Study the drawing (mm; zero at the part's minimum x, y, z) and answer. Coordinates: 2 decimals unless noted, no trailing zeros. Loops run counter-clockwise (first coordinate to the right, second up) from the corner with the lowest first, then second, coordinate; pieces in that order, holes last. Notation, with made-up numbers: (53.25, 40.5) -> (69.25, 40.5) arc R19 cw to (69.25, 50.5) -> close; hole circle Ø6 at (-4, 55). An arc over 180 degrees is marked (long way). One line per question, with ' | ' between items.
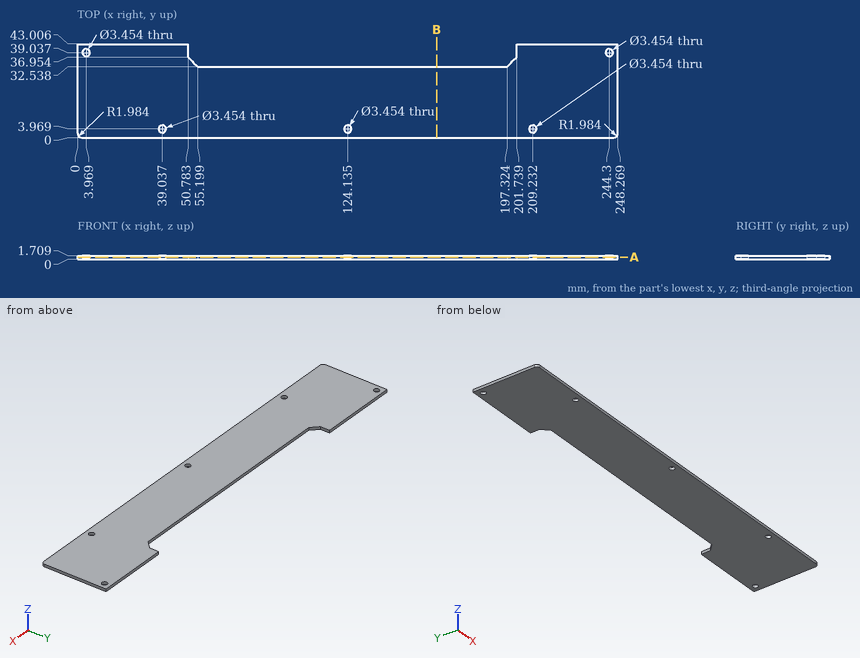
1) A flat-ended cylindrical pin translates along its axis: pin 1 (0.5 mm diameter, centred on x = 134, z = 1, fed in from +Y). Find the tip coordinate at first contact, or state that the pin passes through.
Check values:
pin 1: stops at y = 32.54
2) Find the intervals of material crossed by line 1 along X through (y, z) = (37, 0.8); line 2 along X through (y, z) = (38.5, 0.15); line 3 along Y through (x, z) = (102, 1.25), in increasing order.
Check values:
line 1: x = 0 to 50.78, 201.74 to 248.27 | line 2: x = 0 to 2.33, 5.61 to 50.78, 201.74 to 242.66, 245.94 to 248.27 | line 3: y = 0 to 32.54
3) Find section B-B (x = 165). Write down the section's boundary in (y, z).
Check values:
outline: (0, 0) -> (32.54, 0) -> (32.54, 1.71) -> (0, 1.71) -> close
4) Find section A-A (z = 1). Write down the section's boundary in (x, y) (1 decimal).
Check values:
outline: (0, 2) arc R2 ccw to (2, 0) -> (246.3, 0) arc R2 ccw to (248.3, 2) -> (248.3, 43) -> (201.7, 43) -> (201.7, 37) -> (197.3, 32.5) -> (55.2, 32.5) -> (50.8, 37) -> (50.8, 43) -> (0, 43) -> close; hole circle Ø3.5 at (4, 39); hole circle Ø3.5 at (39, 4); hole circle Ø3.5 at (124.1, 4); hole circle Ø3.5 at (209.2, 4); hole circle Ø3.5 at (244.3, 39)
